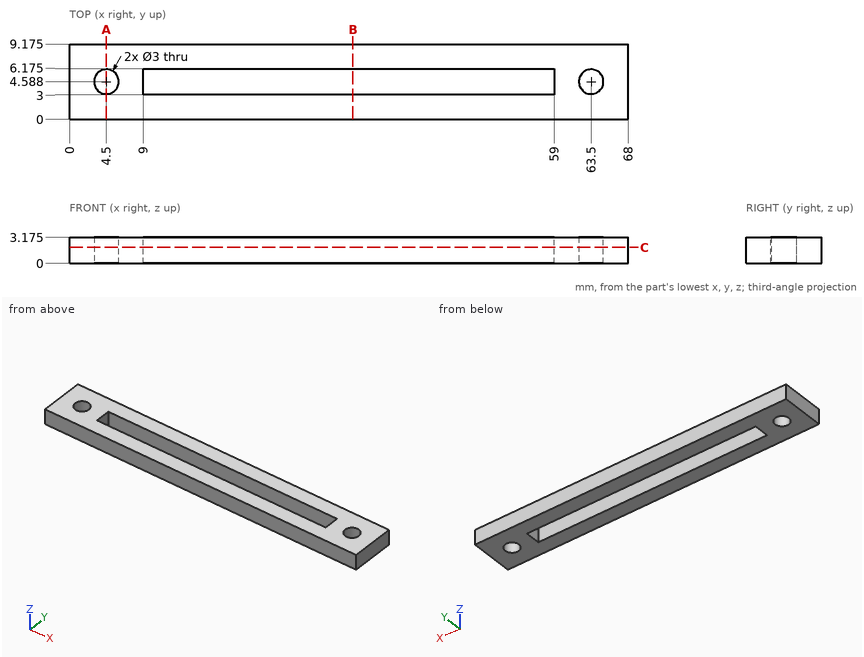
Geometry: see drawing. Coordinates: mm, zero at the bounding-box minimum. Coordinates: 2 decimals unless noted, no trailing zeros. Order: outer loops, then holes, each group sorted by start corner. A loop starts at its lowest first (then second) coordinate and runs counter-clockwise, first axis right, second up. Notation, with made-up numbers: (4, -6) - (42, -6) arc R9 ccw to (42, -1) - close; hole circle Ø11 at (2, 89.5). An arc over 180 degrees is marked (long way). Write each question's results on one line, items separated by ' | '.
1) Section C-C, the plane z = 1.95. Return loops of the section in (x, y) (1 decimal).
Results list:
outline: (0, 0) - (68, 0) - (68, 9.2) - (0, 9.2) - close; hole circle Ø3 at (4.5, 4.6); hole (9, 3) - (59, 3) - (59, 6.2) - (9, 6.2) - close; hole circle Ø3 at (63.5, 4.6)
2) Section B-B, the plane x = 34.5. Return loops of the section in (y, z) (1 decimal).
Results list:
outline: (0, 0) - (3, 0) - (3, 3.2) - (0, 3.2) - close; (6.2, 0) - (9.2, 0) - (9.2, 3.2) - (6.2, 3.2) - close
3) Section A-A, the plane x = 4.5. Return loops of the section in (y, z) (1 decimal), plus the area to 3 significant figures.
Results list:
outline: (0, 0) - (3.1, 0) - (3.1, 3.2) - (0, 3.2) - close; (6.1, 0) - (9.2, 0) - (9.2, 3.2) - (6.1, 3.2) - close | area: 19.6 mm^2
4) Line query: line 1 (Y direction, x = 43, z = 0.8) (1 decimal); line 2 (X direction, y = 4.5, z = 0.2); line 3 (Y direction, x = 4.5, z = 1.3) (1 decimal). Output: solid intervals per line, ascending. Write a range as from..to.
Results list:
line 1: 0..3, 6.2..9.2 | line 2: 0..3, 6..9, 59..62, 65..68 | line 3: 0..3.1, 6.1..9.2
5) Pin query (flat end, axial travel): pin 1 (2.5 mm diameter, centred on x = 4.5, y = 4.59, fed in from -Z). Return the tip coordinate at first contact, or that it passes through.
Results list:
pin 1: through
